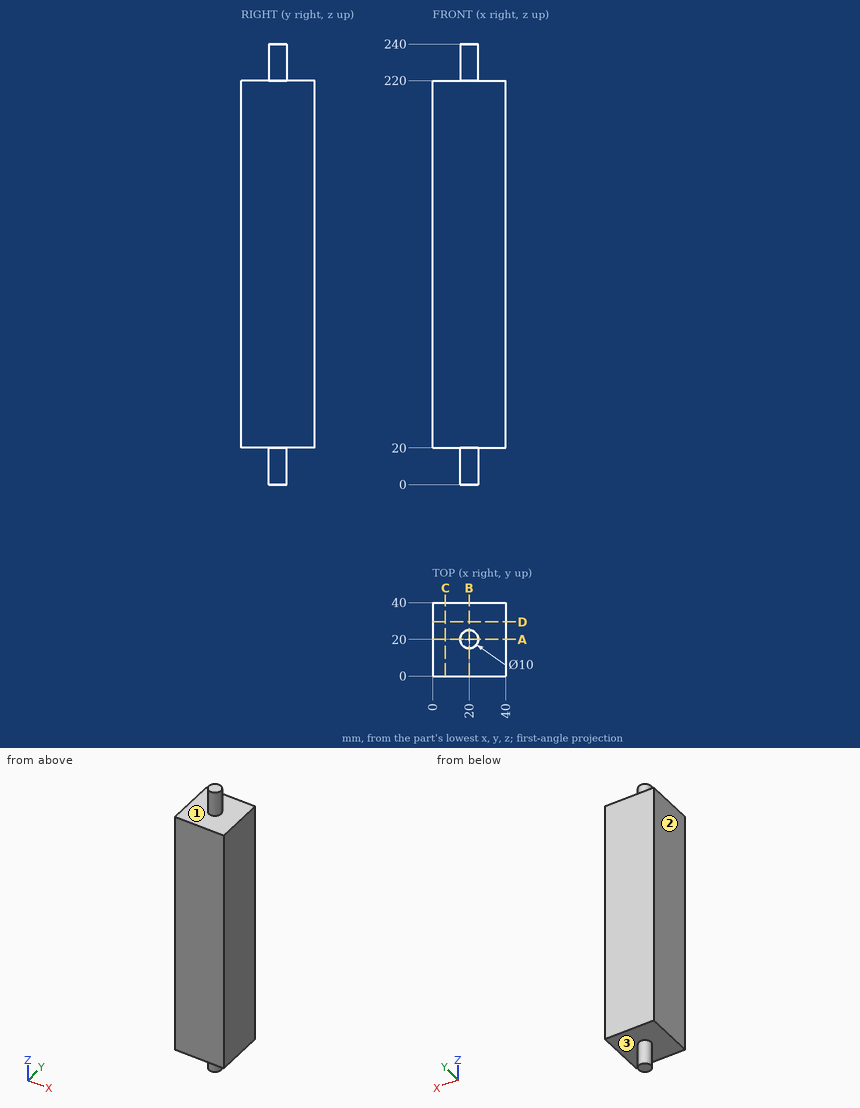
The drawing under review shows one solid part. Ordinate dimensions are in mm from its lowest x, y, z. A direction names the side the tool comes from. Round coordinates to 2 decimals unless told otherwise and drop trailing zeros. Loops run counter-clockwise (first coordinate to the right, second up) from the corner with the lowest first, then second, coordinate; pieces in that order, holes last. Notation, with made-up numbers: M 17.5,21 L 40.5,21 A21 cw 40.5,60 Z; hole C 82,-28 d8. An arc over 180 degrees is marked long. Answer as CSV lines item,"result". Start each with the question number.
Item 1: For the marked faces 1, 2 and 3, list the 3-axis set-ups (+Z, -Z, +X, -X, +Y, -Y) from which the entire face can be reached by the end or side of a thin tool; tool diameter is ignored.
Item 2: Insertion check: P1, Ø12, axis at x = 12.5, y = 29, coming from the +Z side; P2, Ø8, axis at x = 5, y = 14.5, coming from the -Z side. Each pin has a flat end and moves straight along its axis. Give the tip position at first contact, or say it passes through.
Item 3: Consider section A-A (y = 20). Write out the cut boundary in (x, z), then the cut area to 3 significant figures.
Item 4: Wall thickness on line 1 (Z direction, x = 23, y = 28); line 2 (Y direction, x = 23.5, z = 229.5); line 3 (X direction, y = 18, z = 225.5): over which ranges is each line inside the solid? List them lowest first. Write a range as [from, to].
Item 5: Consider section C-C (x = 7). Write out the cut boundary in (y, z), then the cut area to 3 significant figures.
Answer:
1,face 1,"+Z"
1,face 2,"+Z, -Z, -X, +Y, -Y"
1,face 3,"-Z"
2,P1,"stops at z = 220"
2,P2,"stops at z = 20"
3,outline,"M 0,20 L 15,20 L 15,0 L 25,0 L 25,20 L 40,20 L 40,220 L 25,220 L 25,240 L 15,240 L 15,220 L 0,220 Z"
3,area,"8,400 mm^2"
4,line 1,"z = [20, 220]"
4,line 2,"y = [16.43, 23.57]"
4,line 3,"x = [15.42, 24.58]"
5,outline,"M 0,20 L 40,20 L 40,220 L 0,220 Z"
5,area,"8,000 mm^2"
